Design review of the part built by this model. Coordinates are the model's own, in mm. Round coordinates to 2 decimals unless told otherwise and drop trailing zeros. Order: outer loops, then holes, each group sorted by start corner. A loop starts at its lowest first (then second) coordinate and runs counter-clockwise, first axis right, second up. Notation, with made-up numbers: M -6.75,51.25 L 29.25,51.25 A18 cw 29.25,77.25 Z; hole C 42.25,62 d10. An arc over 180 degrees is marked long. Use a Markdown table: item, result. Add a question column.
(1) Take a section at B-B (x = 3.25). Write out the cut boundary in (y, z).
(2) The part is to be moulded in two halves that separate along Y. For faces 1 (the face through (7.493, -0.004, 18.982)), 2 (the face through (7.493, -16.441, 9.488)), 3 (the face through (0, 2.3, -12.2)), say which applies: released by +Y, released by -Y, zero draft, split by the parting line, or undercut.
(3) For pin 1 (13.5 mm diameter, centred on y = 0, z = 0, fed in from -X), flat-tipped, find the tip position at first contact; note if it passes through.
(4) Take a section at D-D (z = -15). Write out the cut boundary in (x, y).
(5) Take a section at C-C (y = -13). Write out the cut boundary in (x, z).
(6) Take a section at A-A (z = 0). Write out the cut boundary in (x, y), then the cut area to 3 significant figures.
(7) To check wall thickness, follow probe 1 along Y at (x, z) = (4.15, 0); probe 2 along Z at (x, y) = (2.7, 0); probe 3 along Z at (x, y) = (5.5, -4). State the ranges of each line that lie inside material, in increasing order. Write a range as from..to.
Autodesk Inventor part; units mm, degrees
ref_plane "YZ Plane" through (0, 0, 0) normal (1, 0, 0) x (0, 1, 0)
ref_plane "XZ Plane" through (0, 0, 0) normal (0, 1, 0) x (-1, 0, 0)
ref_plane "XY Plane" through (0, 0, 0) normal (0, 0, 1) x (1, 0, 0)
sketch "Boceto1" plane through (0, 0, 0) normal (1, 0, 0) x (0, 1, 0)
  line L0 (17, 9.815) -> (17, -9.815)
  line L1 (17, 9.815) -> (0, 0) construction
  line L2 (0, 0) -> (17, -9.815) construction
  line L3 (0, 0) -> (17, 9.815) construction
  line L4 (0, 19.6299) -> (17, 9.815)
  line L5 (0, 19.6299) -> (0, 0) construction
  line L6 (0, 0) -> (0, 19.6299) construction
  line L7 (-17, 9.815) -> (0, 19.6299)
  line L8 (-17, 9.815) -> (0, 0) construction
  line L9 (0, 0) -> (-17, 9.815) construction
  line L10 (-17, -9.815) -> (-17, 9.815)
  line L11 (-17, -9.815) -> (0, 0) construction
  line L12 (0, 0) -> (-17, -9.815) construction
  line L13 (0, -19.6299) -> (-17, -9.815)
  line L14 (0, -19.6299) -> (0, 0) construction
  line L15 (0, 0) -> (0, -19.6299) construction
  line L16 (17, -9.815) -> (0, -19.6299)
  line L17 (17, -9.815) -> (0, 0) construction
  point P0 (17, 0)
  point P1 (8.5, 14.7224)
  point P2 (-8.5, 14.7224)
  point P3 (-17, 0)
  point P4 (-8.5, -14.7224)
  point P5 (8.5, -14.7224)
  point P6 (17, 9.815)
  point P7 (0, 19.6299)
  point P8 (-17, 9.815)
  point P9 (-17, -9.815)
  point P10 (0, -19.6299)
  point P11 (17, -9.815)
  dimension "d1" = 60
  dimension "d2" = 17
  dimension "d5" = 360
extrude "Extrusión1" add sketch "Boceto1" along normal blind 8
hole "Agujero1" at (0, 0, 0) direction (1, 0, 0) diameter 22.3762 end through all
fillet "Empalme1" radius 1 6 edges at (4, 17, -9.815) (4, 0, -19.6299) (4, -17, -9.815) (4, 17, 9.815) (4, 0, 19.6299) (4, -17, 9.815)
chamfer "Chaflán1" distance 1 angle 45 24 edges at (8, 17, 0) (8, 16.866, 9.7376) (8, 8.5, 14.7224) (8, 0, 19.4752) (8, -8.5, 14.7224) (8, -16.866, 9.7376) (8, -17, 0) (8, -16.866, -9.7376) (8, -8.5, -14.7224) (8, 0, -19.4752) (8, 8.5, -14.7224) (8, 16.866, -9.7376) (0, 17, 0) (0, 16.866, 9.7376) (0, 8.5, 14.7224) (0, 0, 19.4752) (0, -8.5, 14.7224) (0, -16.866, 9.7376) (0, -17, 0) (0, -16.866, -9.7376) (0, -8.5, -14.7224) (0, 0, -19.4752) (0, 8.5, -14.7224) (0, 16.866, -9.7376)
chamfer "Chaflán2" distance 1 angle 45 2 edges at (0, 0, -11.1881) (8, 0, -11.1881)
properties part number "tuerca"
Verdict:
| question | item | result |
|---|---|---|
| 1 | outline | M -17,-9.24 A1 ccw -16.5,-10.1 L -0.5,-19.34 A1 ccw 0.5,-19.34 L 16.5,-10.1 A1 ccw 17,-9.24 L 17,9.24 A1 ccw 16.5,10.1 L 0.5,19.34 A1 ccw -0.5,19.34 L -16.5,10.1 A1 ccw -17,9.24 Z; hole C 0,0 d22.38 |
| 2 | face 1 | split by the parting line |
| 2 | face 2 | released by -Y |
| 2 | face 3 | zero draft |
| 3 | pin 1 | passes through |
| 4 | outline | M 0,-6.02 L 1,-8.02 L 7,-8.02 L 8,-6.02 L 8,6.02 L 7,8.02 L 1,8.02 L 0,6.02 Z |
| 5 | outline | M 0,-10.97 L 1,-12.12 L 7,-12.12 L 8,-10.97 L 8,10.97 L 7,12.12 L 1,12.12 L 0,10.97 Z |
| 6 | outline | M 0,-16 L 1,-17 L 7,-17 L 8,-16 L 8,-12.19 L 7,-11.19 L 1,-11.19 L 0,-12.19 Z; M 0,12.19 L 1,11.19 L 7,11.19 L 8,12.19 L 8,16 L 7,17 L 1,17 L 0,16 Z |
| 6 | area | 89.0 mm^2 |
| 7 | probe 1 | y = -17..-11.19, 11.19..17 |
| 7 | probe 2 | z = -19.48..-11.19, 11.19..19.48 |
| 7 | probe 3 | z = -17.32..-10.45, 10.45..17.32 |
